Geometry check sheet. Reference: the model listing, model coordinates, mm. Round coordinates to 2 decimals unless told otherwise and drop trailing zeros. Order: outer loops, then holes, each group sorted by start corner. A loop starts at its lowest first (then second) coordinate and runs counter-clockwise, first axis right, second up. Notation, with made-up numbers: (70.5, 56) - (116.5, 56) arc R38 cw to (116.5, 94) - close; hole circle Ø11 at (18, -13.75). An arc over 180 degrees is marked (long way). One line per question, with ' | ' between items. Start each with the question number.
Q1. Sectioned sample at D-D, the plane x = 116. Enter the section's corners in (y, z).
Q2. Mould release check, pull along X, two halves, no side actions. Record for faces 1 (the face through (700.07, -2.8, 282.18)), 2 (the face through (520.585, -2.8, 655.858)), 3 (the face through (521, 200, 482)): +X half, -X half, draft (parallel to the pull), parting line (faces both ways), or undercut.
Q3. Sectioned sample at B-B, the plane y = 56. Enter the section's corners in (x, z), then the cut area to 3 significant figures.
Q4. Sectioned sample at A-A, the plane z = 325. Enter the section's corners in (x, y), then the cut area to 3 significant figures.
Q5. Sectioned sample at C-C, the plane z = 464.5. Enter the section's corners in (x, y), then the cut area to 3 significant figures.
Q6. Material ranges on line 1 along X through (y, z) = (105, 333.5); line 2 along X through (y, z) = (-176, 72.5); line 3 along Z through (x, y) = (496, -180), recorded low to high.
Q7. Gauge pin test, flat ends, axial feed: P1, Ø2, axis at y = -150, z = 541.5, coming from the -X side; P2, Ø4, axis at y = -7, z = 590, coming from the +X side; P3, Ø8, axis at x = 593.5, y = 119.5, coming from the +Z side. Record the tip position at first contact, or that the pin passes through.
```python
from build123d import *

# Parameters (mm, degrees)
F1_DEPTH      = 200
F1_DEPTH_BACK = 200
F2_T1_DEPTH   = 400
F4_DEPTH      = 400


# Not quite as in the source:
# - a fillet or chamfer that OpenCascade refuses, or shapes differently, is made with other operations: its cross-section is extruded or revolved along the edge and cut away or added


with BuildPart() as f1:
    # F0 (on Front) → F1 (new body, two sides)
    with BuildSketch(Plane.XZ) as f1_sk:
        with BuildLine():
            Line((524.5966985083, 646.8509630198), (516.4602606489, 665.1211129634))
            ThreePointArc((516.4602606489, 665.1211129634), (174.8026570637, 397.3412013082), (0, 0))
            Line((0, 0), (20.2946136834, 0))
            ThreePointArc((20.2946136834, 0), (140.429327731, 313.2929945553), (369.9696430546, 558.0297788724))
            ThreePointArc((369.9696430546, 558.0297788724), (661.1169981621, 340.7216012774), (787.2059225715, 0))
            Line((787.2059225715, 0), (807.2493330572, 0))
            ThreePointArc((807.2493330572, 0), (681.631739827, 346.6110161721), (389.7878488942, 571.8800100128))
            ThreePointArc((389.7878488942, 571.8800100128), (455.5312679724, 612.3522202116), (524.5966985083, 646.8509630198))
        make_face()
    extrude(amount=F1_DEPTH)
    extrude(f1_sk.sketch, amount=-F1_DEPTH_BACK)

    # F2: fillet of radius 80 on 1 edges, made by hand

    # F2_s2 → F2_t1 (join)
    with BuildSketch(Plane.XZ.offset(-200)):
        with BuildLine():
            ThreePointArc((524.5965325964, 646.8513269885), (478.0294026942, 580.3882007889), (513.5263540919, 507.4100453379))
            Line((513.5263540919, 507.4100453379), (509.1010667383, 500.7453599443))
            ThreePointArc((509.1010667383, 500.7453599443), (449.6679775139, 535.8272349913), (386.8614602924, 564.434377111))
            Line((386.8614602924, 564.434377111), (385.2964579687, 578.5003277629))
            ThreePointArc((385.2964579687, 578.5003277629), (451.6430451413, 619.3438525513), (521.2782630933, 654.13076976))
            Line((521.2782630933, 654.13076976), (524.5965325964, 646.8513269885))
        make_face()
    extrude(amount=F2_T1_DEPTH)

    # F3 (on face) → F4 (cut, through all)
    with BuildSketch(Plane(origin=(0, 200, 0), x_dir=(-1, 0, 0), z_dir=(0, 1, 0))):
        with BuildLine():
            ThreePointArc((-468.7201479158, 619.5389112196), (-461.0435334952, 548.7124418966), (-502.4630068664, 490.7491225353))
            ThreePointArc((-502.4630068664, 490.7491225353), (-438.1743029198, 528.2452259031), (-369.9696430546, 558.0297788724))
            ThreePointArc((-369.9696430546, 558.0297788724), (-418.3179553497, 590.4330572448), (-468.7201479158, 619.5389112196))
        make_face()
    extrude(amount=-F4_DEPTH, mode=Mode.SUBTRACT)


solid = f1.part
```
Determined:
1) outline: (-200, 271.8) - (200, 271.8) - (200, 311.76) - (-200, 311.76) - close
2) face 1: undercut | face 2: +X half | face 3: draft
3) outline: (0, 0) - (20.29, 0) arc R872 cw to (468.72, 619.54) arc R100 ccw to (502.46, 490.75) arc R640.43 cw to (787.21, 0) - (807.25, 0) arc R660.43 ccw to (513.33, 507.54) arc R80 cw to (524.56, 646.83) arc R872 cw to (524.6, 646.85) - (516.46, 665.12) arc R892 ccw to start | area: 32,200 mm2
4) outline: (124.16, -200) - (147.9, -200) - (147.9, 200) - (124.16, 200) - close; (672.5, -200) - (696.76, -200) - (696.76, 200) - (672.5, 200) - close | area: 19,200 mm2
5) outline: (232.52, -200) - (260.39, -200) - (260.39, 200) - (232.52, 200) - close; (539.13, -200) - (571.1, -200) - (571.1, 200) - (539.13, 200) - close | area: 23,900 mm2
6) line 1: x = 129.57 to 153.48, 666.44 to 690.96 | line 2: x = 15.47 to 36.14, 778.18 to 798.5 | line 3: z = 495.42 to 523.23, 624.88 to 655.7
7) P1: stops at x = 314.32 | P2: stops at x = 479.82 | P3: stops at z = 448.57
